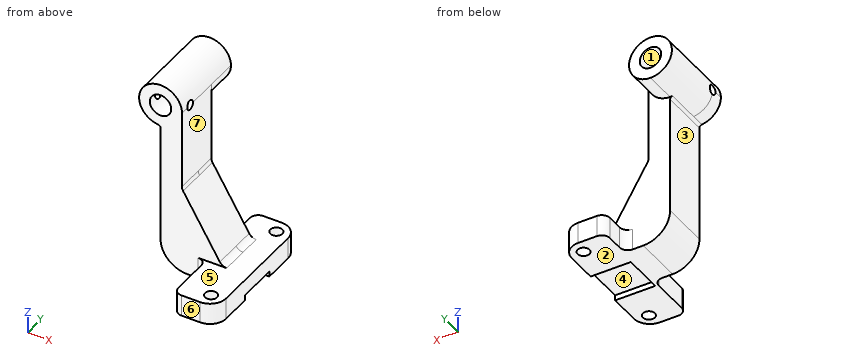
from build123d import *

# Parameters (mm, degrees)
SKETCH_6_R               = 4
EXTRUDE_3_DEPTH          = 25
FILLET_1_R               = 10
FILLET_2_R               = 3
SKETCH_7_R               = 2.25
CUT_EXTRUDE_4_DEPTH      = 50
SKETCH_8_R               = 1.75
CUT_EXTRUDE_5_DEPTH      = 50
EXTRUDE_4_DEPTH          = 5
FILLET_5_R               = 3
FILLET_6_R               = 6
SKETCH_11_W              = 55
SKETCH_11_H              = 12
CUT_EXTRUDE_7_DEPTH      = 17
CUT_EXTRUDE_8_DEPTH      = 80.214897752
CUT_EXTRUDE_8_DEPTH_BACK = 80.214897752
SKETCH_12_W              = 30.277816987
SKETCH_12_H              = 21.642627305
FILLET_7_R               = 8
FILLET_8_R               = 3
FILLET_9_R               = 1
FILLET_10_R              = 3
EXTRUDE_5_DEPTH          = 8
SKETCH_14_W              = 30
SKETCH_14_H              = 15
CUT_EXTRUDE_9_DEPTH      = 2


with BuildPart() as part:
    # 草图6 → 凸台-拉伸3 (new, symmetric)
    with BuildSketch(Plane(origin=(0, 0, 0), x_dir=(1, 0, 0), z_dir=(0, 1, 0))):
        with BuildLine():
            Line((0, 0), (-25, 0))
            Line((-25, 0), (-25, -55))
            ThreePointArc((-25, -55), (-33, -63), (-41, -55))
            ThreePointArc((-41, -55), (-38.656854249, -49.343145751), (-33, -47))
            Line((-33, -47), (-33, 8))
            Line((-33, 8), (0, 8))
            Line((0, 8), (0, 0))
        make_face()
        with Locations(Location((-33, -55, 0), (0, 0, 270))):
            Circle(SKETCH_6_R, mode=Mode.SUBTRACT)
    extrude(amount=EXTRUDE_3_DEPTH, both=True)

    # 圆角1
    fillet_1_edges = [part.edges().sort_by_distance(p)[0] for p in [
        (-33, 0, -8),
    ]]
    fillet(fillet_1_edges, radius=FILLET_1_R)

    # 圆角2
    fillet_2_edges = [part.edges().sort_by_distance(p)[0] for p in [
        (-25, 0, 0),
    ]]
    fillet(fillet_2_edges, radius=FILLET_2_R)

    # 草图7 → 切除-拉伸4 (cut)
    with BuildSketch(Plane(origin=(0, 0, -8), x_dir=(-1, 0, 0), z_dir=(0, 0, -1))):
        with Locations((5, 20)):
            Circle(SKETCH_7_R)
        with Locations((5, -20)):
            Circle(SKETCH_7_R)
    extrude(amount=-CUT_EXTRUDE_4_DEPTH, mode=Mode.SUBTRACT)

    # 草图8 → 切除-拉伸5 (cut)
    with BuildSketch(Plane(origin=(-25, 0, 0), x_dir=(0, 0, -1), z_dir=(1, 0, 0))):
        with Locations((-55, 0)):
            Circle(SKETCH_8_R)
    extrude(amount=-CUT_EXTRUDE_5_DEPTH, mode=Mode.SUBTRACT)

    # 草图9 → 凸台-拉伸4 (add, symmetric)
    with BuildSketch(Plane(origin=(0, 0, 0), x_dir=(1, 0, 0), z_dir=(0, 1, 0))):
        with BuildLine():
            Line((-10, 0), (-25, -25))
            Line((-25, -25), (-25, -3))
            ThreePointArc((-25, -3), (-24.121320344, -0.878679656), (-22, 0))
            Line((-22, 0), (-10, 0))
        make_face()
    extrude(amount=EXTRUDE_4_DEPTH, both=True)

    # 圆角5
    fillet_5_edges = [part.edges().sort_by_distance(p)[0] for p in [
        (-10, 0, 0),
        (-25, 0, 25),
    ]]
    fillet(fillet_5_edges, radius=FILLET_5_R)

    # 圆角6
    fillet_6_edges = [part.edges().sort_by_distance(p)[0] for p in [
        (0, 25, -4),
        (0, -25, -4),
    ]]
    fillet(fillet_6_edges, radius=FILLET_6_R)

    # 草图11 → 切除-拉伸7 (cut)
    with BuildSketch(Plane.ZY.offset(33)):
        with Locations((19.5, 19)):
            Rectangle(SKETCH_11_W, SKETCH_11_H)
        with Locations((19.5, -19)):
            Rectangle(SKETCH_11_W, SKETCH_11_H)
    extrude(amount=-CUT_EXTRUDE_7_DEPTH, mode=Mode.SUBTRACT)

    # 草图12 → 切除-拉伸8 (cut, two sides: drawn at the far end of the back side and taken through both)
    with BuildSketch(Plane.XY.offset(-CUT_EXTRUDE_8_DEPTH_BACK)):
        with Locations((-31.138908494, -15.821313653)):
            Rectangle(SKETCH_12_W, SKETCH_12_H)
    extrude(amount=CUT_EXTRUDE_8_DEPTH + CUT_EXTRUDE_8_DEPTH_BACK, mode=Mode.SUBTRACT)

    # 圆角7
    fillet_7_edges = [part.edges().sort_by_distance(p)[0] for p in [
        (-25, 19, 47),
    ]]
    fillet(fillet_7_edges, radius=FILLET_7_R - 0.0001)  # a hair under: the kernel refuses the full size

    # 圆角8
    fillet_8_edges = [part.edges().sort_by_distance(p)[0] for p in [
        (-16, 13, -4),
        (-16, 25, -4),
    ]]
    fillet(fillet_8_edges, radius=FILLET_8_R)

    # 圆角9
    fillet_9_edges = [part.edges().sort_by_distance(p)[0] for p in [
        (-33, 6.5, 47),
    ]]
    fillet(fillet_9_edges, radius=FILLET_9_R)

    # 圆角10
    fillet_10_edges = [part.edges().sort_by_distance(p)[0] for p in [
        (-16, -25, -4),
        (-16, -5, -4),
    ]]
    fillet(fillet_10_edges, radius=FILLET_10_R)

    # 草图13 → 凸台-拉伸5 (add)
    with BuildSketch(Plane(origin=(0, 5, 0), x_dir=(1, 0, 0), z_dir=(0, 1, 0))):
        with BuildLine():
            Line((-8.301428863, 0), (-22, 0))
            ThreePointArc((-22, 0), (-24.121320344, -0.878679656), (-25, -3))
            Line((-25, -3), (-25, -25.830951895))
            ThreePointArc((-25, -25.830951895), (-24.891144785, -25.030151149), (-24.572478777, -24.287464629))
            Line((-24.572478777, -24.287464629), (-10.87390764, -1.456512734))
            ThreePointArc((-10.87390764, -1.456512734), (-9.779525308, -0.38940028), (-8.301428863, 0))
        make_face()
    extrude(amount=EXTRUDE_5_DEPTH)

    # 草图14 → 切除-拉伸9 (cut)
    with BuildSketch(Plane(origin=(0, 0, -8), x_dir=(-1, 0, 0), z_dir=(0, 0, -1))):
        Rectangle(SKETCH_14_W, SKETCH_14_H)
    extrude(amount=-CUT_EXTRUDE_9_DEPTH, mode=Mode.SUBTRACT)


solid = part.part
Can you work these out from the model? Positions are in its coordinate system, mm. Face numbers are marked on the shaded views. A direction names the side the tool comes from. Give positions to 0.01 mm unless a question says otherwise; leave off trailing zeros. Order: outer loops, then holes, each group sorted by start corner. A loop starts at its lowest first (then second) coordinate and runs counter-clockwise, first axis right, second up. Notation, with made-up numbers: M 59.25,77.25 L 101.25,77.25 A23 cw 101.25,94.25 Z; hole C -32,-14.5 d10. An arc over 180 degrees is marked long. Use one line per item in the form item = value.
Item 1: If we section it at B-B, the plane x = -5: Write out the boundary of the cut face in (y, z), and give its area (3 significant figures).
Values follow:
outline = M -24.92,-8 L -22.25,-8 L -22.25,0 L -24.92,0 Z; M -17.75,-8 L -7.5,-8 L -7.5,-6 L 7.5,-6 L 7.5,-8 L 17.75,-8 L 17.75,0 L -17.75,0 Z; M 22.25,-8 L 24.92,-8 L 24.92,0 L 22.25,0 Z
area = 297 mm^2
Item 2: Thinking about a two-plate mould opening in X: for the marked faces 1, 2 and 3, which applies, pulls with the +X half, pulls with the -X half, needs draft (parallel to the pull), parting line crosses it, or undercut?
Values follow:
face_1 = undercut
face_2 = needs draft
face_3 = pulls with the -X half
Item 3: If I drill on line 1 along X through (y, z) = (7, 55); line 2 along Z through (x, y) = (-33, 16.5); line 3 along Y through (x, z) = (-5, -5), over which ranges is the centre line in solid material (lowest first)? Write a range as [from, to].
Values follow:
line_1 = [-41, -37], [-29, -25]
line_2 = [47, 51], [59, 63]
line_3 = [-24.92, -22.25], [-17.75, 17.75], [22.25, 24.92]
Item 4: For the marked faces 4, 5, 6 and 7, which set-ups out of +Z, -Z, +X, -X, +Y, -Y let a thin tool reach every point of the face, with its end or its side?
Values follow:
face_4 = -Z, +X
face_5 = +Z, +X
face_6 = +Z, -Z, +X, -X, -Y
face_7 = +Z, +X, +Y, -Y
Item 5: Will these pins go through, and if not, where does the flat tip stop? pin 1 Ø6 at (x, z) = (-9, 3.5) entering from +Y; pin 2 Ø9 at (y, z) = (3, 22) entering from -X; pin 3 Ø4 at (y, z) = (-18, -2) entering from -X; pin 4 Ø3.5 at (x, y) = (-5, -20) entering from -Z.
Values follow:
pin_1 = 13
pin_2 = -33
pin_3 = -16
pin_4 = through
Item 6: If we section it at A-A, the plane y = 10: Write out the boundary of the cut face in (x, z), and give its area (3 significant figures).
Values follow:
outline = M -33.89,47.05 A1 cw -33,46.06 L -33,2 A10 ccw -23,-8 L 0,-8 L 0,0 L -8.3,0 A3 cw -10.87,1.46 L -24.57,24.29 A3 cw -25,25.83 L -25,55 A8 ccw long Z; hole C -33,55 d8
area = 971 mm^2
Item 7: If we section it at C-C, the plane z = -1.5: Write out the boundary of the cut face in (x, y), and give its area (3 significant figures).
Values follow:
outline = M -32.37,-5 L -19,-5 A3 cw -16,-8 L -16,-22 A3 ccw -13,-25 L -6,-25 A6 ccw 0,-19 L 0,19 A6 ccw -6,25 L -13,25 A3 ccw -16,22 L -16,16 A3 cw -19,13 L -32.37,13 Z; hole C -5,-20 d4.5; hole C -5,20 d4.5
area = 1,050 mm^2
Item 8: If we section it at D-D, the plane y = -20: Write out the boundary of the cut face in (x, z).
Values follow:
outline = M -16,-8 L -7.25,-8 L -7.25,0 L -16,0 Z; M -2.75,-8 L -0.08,-8 L -0.08,0 L -2.75,0 Z
